from build123d import *

# Parameters (mm, degrees)
SKETCH1_W            = 57.7
SKETCH1_H            = 114.7
BOSS_EXTRUDE1_DEPTH  = 3
SKETCH2_R            = 1.6
CUT_EXTRUDE1_DEPTH   = 3
CHAMFER1_SIZE        = 2
CHAMFER1_SIZE2       = 1.678199262
SKETCH4_W            = 57.7
SKETCH4_H            = 3
BOSS_EXTRUDE2_DEPTH  = 1.6
SKETCH5_W            = 19
SKETCH5_H            = 6
BOSS_EXTRUDE3_DEPTH  = 2.2
SKETCH7_W            = 19
SKETCH7_H            = 3
BOSS_EXTRUDE4_DEPTH  = 4.5
CHAMFER2_SIZE        = 0.5
SKETCH8_W            = 25.7
SKETCH8_H            = 3
SKETCH8_W_2          = 25
SKETCH8_H_2          = 4
BOSS_EXTRUDE5_DEPTH  = 2
SKETCH9_W            = 25.7
SKETCH9_H            = 7
BOSS_EXTRUDE6_DEPTH  = 4.5
SKETCH10_R           = 2
CUT_EXTRUDE2_DEPTH   = 3
SKETCH11_W           = 4
SKETCH11_H           = 2
BOSS_EXTRUDE7_DEPTH  = 0.7
SKETCH12_W           = 4
SKETCH12_H           = 1.993871031
SKETCH12_H_2         = 2
BOSS_EXTRUDE11_DEPTH = 0.7
SKETCH13_W           = 4.5
SKETCH13_H           = 3
SKETCH13_W_2         = 3
BOSS_EXTRUDE12_DEPTH = 2
SKETCH14_W           = 2.5
SKETCH14_H           = 10
BOSS_EXTRUDE13_DEPTH = 2
CHAMFER3_SIZE        = 1


with BuildPart() as part:
    # Sketch1 → Boss-Extrude1 (new body)
    with BuildSketch(Plane.XY):
        with Locations((28.85, 57.35)):
            Rectangle(SKETCH1_W, SKETCH1_H)
    extrude(amount=BOSS_EXTRUDE1_DEPTH)

    # Sketch2 → Cut-Extrude1 (cut)
    with BuildSketch(Plane.XY.offset(3)):
        with Locations((5.3, 109.4)):
            Circle(SKETCH2_R)
        with Locations((52.4, 109.4)):
            Circle(SKETCH2_R)
        with Locations((9.85, 4.2)):
            Circle(SKETCH2_R)
        with Locations((45.9, 4.2)):
            Circle(SKETCH2_R)
    extrude(amount=-CUT_EXTRUDE1_DEPTH, mode=Mode.SUBTRACT)

    # Chamfer1
    chamfer1_edges = [part.edges().sort_by_distance(p)[0] for p in [
        (3.7, 109.4, 3),
        (44.3, 4.2, 3),
        (8.25, 4.2, 3),
        (50.8, 109.4, 3),
    ]]
    chamfer1_side = [part.faces().sort_by_distance(p)[0] for p in [
        (28.85238123, 57.352686516, 3),
    ]]
    chamfer(chamfer1_edges, length=CHAMFER1_SIZE, length2=CHAMFER1_SIZE2, reference=chamfer1_side[0])

    # Sketch4 → Boss-Extrude2 (add)
    with BuildSketch(Plane.XZ):
        with Locations((28.85, 1.5)):
            Rectangle(SKETCH4_W, SKETCH4_H)
    extrude(amount=BOSS_EXTRUDE2_DEPTH)

    # Sketch5 → Boss-Extrude3 (add)
    with BuildSketch(Plane(origin=(0, 0, 0), x_dir=(-1, 0, 0), z_dir=(0, 0, -1))):
        with Locations((-36.2, 102.2)):
            Rectangle(SKETCH5_W, SKETCH5_H)
    extrude(amount=BOSS_EXTRUDE3_DEPTH)

    # Sketch7 → Boss-Extrude4 (add)
    with BuildSketch(Plane(origin=(0, 0, 0), x_dir=(-1, 0, 0), z_dir=(0, 0, -1))):
        with Locations((-36.2, 105.7)):
            Rectangle(SKETCH7_W, SKETCH7_H)
    extrude(amount=BOSS_EXTRUDE4_DEPTH)

    # Chamfer2
    chamfer2_edges = [part.edges().sort_by_distance(p)[0] for p in [
        (36.2, 104.2, -4.5),
    ]]
    chamfer(chamfer2_edges, length=CHAMFER2_SIZE)

    # Sketch8 → Boss-Extrude5 (add)
    with BuildSketch(Plane(origin=(0, 0, 0), x_dir=(-1, 0, 0), z_dir=(0, 0, -1))):
        with Locations((-26.85, 27.9)):
            Rectangle(SKETCH8_W, SKETCH8_H)
        with Locations((-42.2, 33.4)):
            Rectangle(SKETCH8_W_2, SKETCH8_H_2)
    extrude(amount=BOSS_EXTRUDE5_DEPTH)

    # Sketch9 → Boss-Extrude6 (add)
    with BuildSketch(Plane(origin=(0, 0, 0), x_dir=(-1, 0, 0), z_dir=(0, 0, -1))):
        with Locations((-26.85, 13.9)):
            Rectangle(SKETCH9_W, SKETCH9_H)
    extrude(amount=BOSS_EXTRUDE6_DEPTH)

    # Sketch10 → Cut-Extrude2 (cut)
    with BuildSketch(Plane.XY.offset(3)):
        with Locations((53.7, 19.9)):
            Circle(SKETCH10_R)
        with Locations((53.7, 12.4)):
            Circle(SKETCH10_R)
        with Locations((53.7, 4.9)):
            Circle(SKETCH10_R)
    extrude(amount=-CUT_EXTRUDE2_DEPTH, mode=Mode.SUBTRACT)

    # Sketch11 → Boss-Extrude7 (add)
    with BuildSketch(Plane.XY.offset(3)):
        with Locations((53.7, 20.9)):
            Rectangle(SKETCH11_W, SKETCH11_H)
        with Locations((53.7, 13.4)):
            Rectangle(SKETCH11_W, SKETCH11_H)
        with Locations((53.7, 5.9)):
            Rectangle(SKETCH11_W, SKETCH11_H)
    extrude(amount=-BOSS_EXTRUDE7_DEPTH)

    # Sketch12 → Boss-Extrude11 (add)
    with BuildSketch(Plane(origin=(0, 0, 0), x_dir=(-1, 0, 0), z_dir=(0, 0, -1))):
        with Locations((-53.7, 18.903064484)):
            Rectangle(SKETCH12_W, SKETCH12_H)
        with Locations((-53.7, 11.4)):
            Rectangle(SKETCH12_W, SKETCH12_H_2)
        with Locations((-53.7, 3.9)):
            Rectangle(SKETCH12_W, SKETCH12_H_2)
    extrude(amount=-BOSS_EXTRUDE11_DEPTH)

    # Sketch13 → Boss-Extrude12 (add)
    with BuildSketch(Plane(origin=(0, 0, 0), x_dir=(-1, 0, 0), z_dir=(0, 0, -1))):
        with Locations((-53.8, 3.1)):
            Rectangle(SKETCH13_W, SKETCH13_H)
        with Locations((-3.5, 3.1)):
            Rectangle(SKETCH13_W_2, SKETCH13_H)
    extrude(amount=BOSS_EXTRUDE12_DEPTH)

    # Sketch14 → Boss-Extrude13 (add)
    with BuildSketch(Plane(origin=(0, 0, 0), x_dir=(-1, 0, 0), z_dir=(0, 0, -1))):
        with Locations((-54.95, 69.7)):
            Rectangle(SKETCH14_W, SKETCH14_H)
        with Locations((-26.25, 69.7)):
            Rectangle(SKETCH14_W, SKETCH14_H)
    extrude(amount=BOSS_EXTRUDE13_DEPTH)

    # Chamfer3
    chamfer3_edges = [part.edges().sort_by_distance(p)[0] for p in [
        (28.85, -1.6, 3),
    ]]
    chamfer(chamfer3_edges, length=CHAMFER3_SIZE)


solid = part.part
Part model, mm, in its own coordinate system. A direction names the side the tool comes from. Give positions to 0.01 mm unless a question says otherwise; leave off trailing zeros. Write each loop counter-clockwise with the first axis right and the second up, starting at its lowest first coordinate (ties: lowest second). Pieces come first, ordered by that corner, then holes.
1) Which spindle directions (+Z, -Z, +X, -X, +Y, -Y) get a long thin tool onto all of the face, cutting with end or side? Do faces 4 (the face through (39.7, 14, -2)), 5 (the face through (27.5, 70, -1)), 6 (the face through (26.7, 104, -2)), 7 (the face through (27, 28, -2)), 8 (the face through (27, 10.4, -2)). Say none if no direction does.
Resolved:
face 4: -Z, +X, -Y
face 5: -Z
face 6: -Z, -X, +Y
face 7: -Z, +X, -X
face 8: -Z, +X, -X, -Y
2) Cut at B-B on x = 19. Write the cut outline in (y, z).
Resolved:
outline: (-1.6, 0) - (10.4, 0) - (10.4, -4.5) - (17.4, -4.5) - (17.4, 0) - (26.4, 0) - (26.4, -2) - (29.4, -2) - (29.4, 0) - (114.7, 0) - (114.7, 3) - (-0.6, 3) - (-1.6, 2) - close
3) Probe L1, parallel to X at y = 109.4, z = 0.65; L2, parallel to Y at x = 29.5, z = -0.25; L3, parallel to Y at x = 36, z = -0.75. List the from-to ranges inside material, lowest first.
Resolved:
L1: x = 0 to 3.7, 6.9 to 50.8, 54 to 57.7
L2: y = 10.4 to 17.4, 26.4 to 29.4, 99.2 to 107.2
L3: y = 10.4 to 17.4, 26.4 to 29.4, 31.4 to 35.4, 99.2 to 107.2
4) Two-plate mould, pull along X, no slides. Class faces 1 (the face through (54, 6, 2.3)), 2 (the face through (27, 29.4, -1)), 3 (the face through (2, 3, -1)): released by +X, released by -X, zero draft, split by the parting line, or undercut.
Resolved:
face 1: undercut
face 2: zero draft
face 3: released by -X
5) Pin check, flat tips, straight feed: pin 1 (1.3 mm diameter, centred on x = 36.5, z = -1.5, fed in from +Y); pin 2 (1 mm diameter, centred on x = 30.5, z = -1, fed in from -Y); pin 3 (1.6 mm diameter, centred on x = 53, z = -1.5, fed in from +Y). Stop position of each tip, or through.
Resolved:
pin 1: stops at y = 107.2
pin 2: stops at y = 10.4
pin 3: stops at y = 74.7
6) Cut at A-A on y = 68.5. Write the cut outline in (x, z).
Resolved:
outline: (0, 0) - (25, 0) - (25, -2) - (27.5, -2) - (27.5, 0) - (53.7, 0) - (53.7, -2) - (56.2, -2) - (56.2, 0) - (57.7, 0) - (57.7, 3) - (0, 3) - close
7) Cut at C-C on y = 16. Write the cut outline in (x, z), then the cut area to 3 significant figures.
Resolved:
outline: (0, 0) - (14, 0) - (14, -4.5) - (39.7, -4.5) - (39.7, 0) - (57.7, 0) - (57.7, 3) - (0, 3) - close
area: 289 mm2
8) Cut at D-D on y = 89. Write the cut outline in (x, z).
Resolved:
outline: (0, 0) - (57.7, 0) - (57.7, 3) - (0, 3) - close
